Autodesk Inventor part; units mm, degrees
ref_plane "YZ Plane" through (0, 0, 0) normal (1, 0, 0) x (0, 1, 0)
ref_plane "XZ Plane" through (0, 0, 0) normal (0, 1, 0) x (-1, 0, 0)
ref_plane "XY Plane" through (0, 0, 0) normal (0, 0, 1) x (1, 0, 0)
sketch "Sketch1" plane through (0, 0, 0) normal (1, 0, 0) x (0, 1, 0)
  line L0 (-9.11, -10.73) -> (9.11, -10.73)
  line L1 (11.11, -8.73) -> (11.11, 8.73)
  line L2 (9.11, 10.73) -> (-9.11, 10.73)
  line L3 (-11.11, 8.73) -> (-11.11, -8.73)
  line L4 (-11.11, -10.73) -> (11.11, 10.73) construction
  line L5 (11.11, -10.73) -> (-11.11, 10.73) construction
  arc A0 (11.11, 8.73) -> (9.11, 10.73) centre (9.11, 8.73) ccw
  arc A1 (9.11, -10.73) -> (11.11, -8.73) centre (9.11, -8.73) ccw
  arc A2 (-11.11, -8.73) -> (-9.11, -10.73) centre (-9.11, -8.73) ccw
  arc A3 (-9.11, 10.73) -> (-11.11, 8.73) centre (-9.11, 8.73) ccw
  point P0 (0, 0)
  dimension "d0" = 22.22
  dimension "d1" = 21.46
  dimension "d2" = 2
extrude "Extrusion1" add sketch "Sketch1" along normal blind 94
sketch "Sketch2" plane through (94, 0, 0) normal (1, 0, 0) x (0, 0, -1)
  line L0 (-6.6347, 7.2513) -> (6.6347, 7.2513)
  line L1 (6.6347, 7.2513) -> (6.6347, 2.4915)
  line L2 (6.6347, 2.4915) -> (-6.6347, 2.4915)
  line L3 (-6.6347, 2.4915) -> (-6.6347, 7.2513)
  line L4 (-6.6347, 7.2513) -> (6.6347, 2.4915) construction
  line L5 (6.6347, 7.2513) -> (-6.6347, 2.4915) construction
  line L6 (-4.3158, -3.8551) -> (4.3158, -3.8551)
  line L7 (4.3158, -3.8551) -> (4.3158, -5.8078)
  line L8 (4.3158, -5.8078) -> (-4.3158, -5.8078)
  line L9 (-4.3158, -5.8078) -> (-4.3158, -3.8551)
  line L10 (-4.3158, -3.8551) -> (4.3158, -5.8078) construction
  line L11 (4.3158, -3.8551) -> (-4.3158, -5.8078) construction
  point P0 (0, 0)
  point P1 (0, 4.8714)
  point P2 (0, -4.8314)
extrude "Extrusion2" cut sketch "Sketch2" against normal blind 3
sketch "Sketch3" plane through (0, -9.11, 10.73) normal (0, 0, 1) x (1, 0, 0)
  line L0 (0, 18.22) -> (0, 0)
  line L1 (0, 0) -> (94, 0)
  line L2 (94, 18.22) -> (94, 0)
  line L3 (0, 18.22) -> (94, 18.22)
  line L4 (71.8, 14.11) -> (80, 14.11)
  line L5 (80, 14.11) -> (80, 4.11)
  line L6 (80, 4.11) -> (71.8, 4.11)
  line L7 (71.8, 4.11) -> (71.8, 14.11)
  line L8 (71.8, 14.11) -> (80, 4.11) construction
  line L9 (80, 14.11) -> (71.8, 4.11) construction
  point P0 (0, 9.11)
  point P1 (75.9, 9.11)
  dimension "d7" = 8.2
  dimension "d8" = 10
  dimension "d9" = 14
extrude "Extrusion3" add sketch "Sketch3" along normal blind 3 contours L4 L5 L6 L7
properties part number "00_Batterypack"
Can you work these out from the model? Positions are in its coordinate system, mm. A direction names the side the tool comes from. Coordinates: 2 decimals unless noted, no trailing zeros. Write each loop counter-clockwise with the first axis right and the second up, starting at its lowest first coordinate (ties: lowest second). Pieces come first, ordered by that corner, then holes. Notation, with made-up numbers: (18, 47) -> (59, 47) arc R16 cw to (59, 65) -> close; hole circle Ø8 at (25, 35.25). An arc over 180 degrees is marked (long way). Write item = value, one per line.
(1) For pin 1 (0.6 mm diameter, centred on y = -5, z = 0.5, fed in from +X); pin 2 (3.5 mm diameter, centred on x = 76, z = 12, fed in from +Y); pin 3 (0.6 mm diameter, centred on x = 93, y = -5, fed in from +Z), each with a flat end and sliding along its axis, tell me the tip position at first contact or that it passes through.
Verdict:
pin_1 = 91
pin_2 = 10.41
pin_3 = 10.73
(2) Imagine slicing it at A-A (x = 17.5). Please give me the cut outline in (y, z), and give its area (3 significant figures).
Verdict:
outline = (-11.11, -8.73) arc R2 ccw to (-9.11, -10.73) -> (9.11, -10.73) arc R2 ccw to (11.11, -8.73) -> (11.11, 8.73) arc R2 ccw to (9.11, 10.73) -> (-9.11, 10.73) arc R2 ccw to (-11.11, 8.73) -> close
area = 473 mm^2
(3) Thinking about a two-plate mould opening in Y: for faces 1 (the face through (46.34, 10.51, 10.16)), 2 (the face through (94, 0, 0)), 3 (the face through (93, -5, -4.316)), which applies, +Y half, -Y half, draft (parallel to the pull), parting line (faces both ways), or undercut?
Verdict:
face_1 = +Y half
face_2 = draft
face_3 = undercut
(4) Imagine slicing it at B-B (z = 12.25). Please give me the cut outline in (x, y).
Verdict:
outline = (71.8, -5) -> (80, -5) -> (80, 5) -> (71.8, 5) -> close
(5) Imagine slicing it at C-C (x = 78). Please give me the cut outline in (y, z), and give its area (3 significant figures).
Verdict:
outline = (-11.11, -8.73) arc R2 ccw to (-9.11, -10.73) -> (9.11, -10.73) arc R2 ccw to (11.11, -8.73) -> (11.11, 8.73) arc R2 ccw to (9.11, 10.73) -> (5, 10.73) -> (5, 13.73) -> (-5, 13.73) -> (-5, 10.73) -> (-9.11, 10.73) arc R2 ccw to (-11.11, 8.73) -> close
area = 503 mm^2
(6) If I drill on probe 1 along Z at (x, y) = (28, -1.5); probe 2 along X at (y, z) = (5.25, -0.75); probe 3 along Z at (x, y) = (74, 10), over which ranges is the centre line in solid material (lowest first)?
Verdict:
probe_1 = -10.73 to 10.73
probe_2 = 0 to 91
probe_3 = -10.52 to 10.52
(7) On a 3-axis mill with a long thin cutter (end or side, diameter ignored), from which of +Z, -Z, +X, -X, +Y, -Y can I reach the whole of each face in a straight line? I mean faces 4 (the face through (93, 5, 6.635)), 5 (the face through (76, -5, 12)), 6 (the face through (71.8, 0, 12)). Say none if no direction works.
Verdict:
face_4 = +X
face_5 = +Z, +X, -X, -Y
face_6 = +Z, -X, +Y, -Y
